Source: three-view drawing plus pictorial views. Frame: mm from the lowest corner of the part. A direction names the side the tool comes from. Give positions to 0.01 mm unless a question says otherwise; leave off trailing zeros. Order: outer loops, then holes, each group sorted by start corner. A loop starts at its lowest first (then second) coordinate and runs counter-clockwise, first axis right, second up.
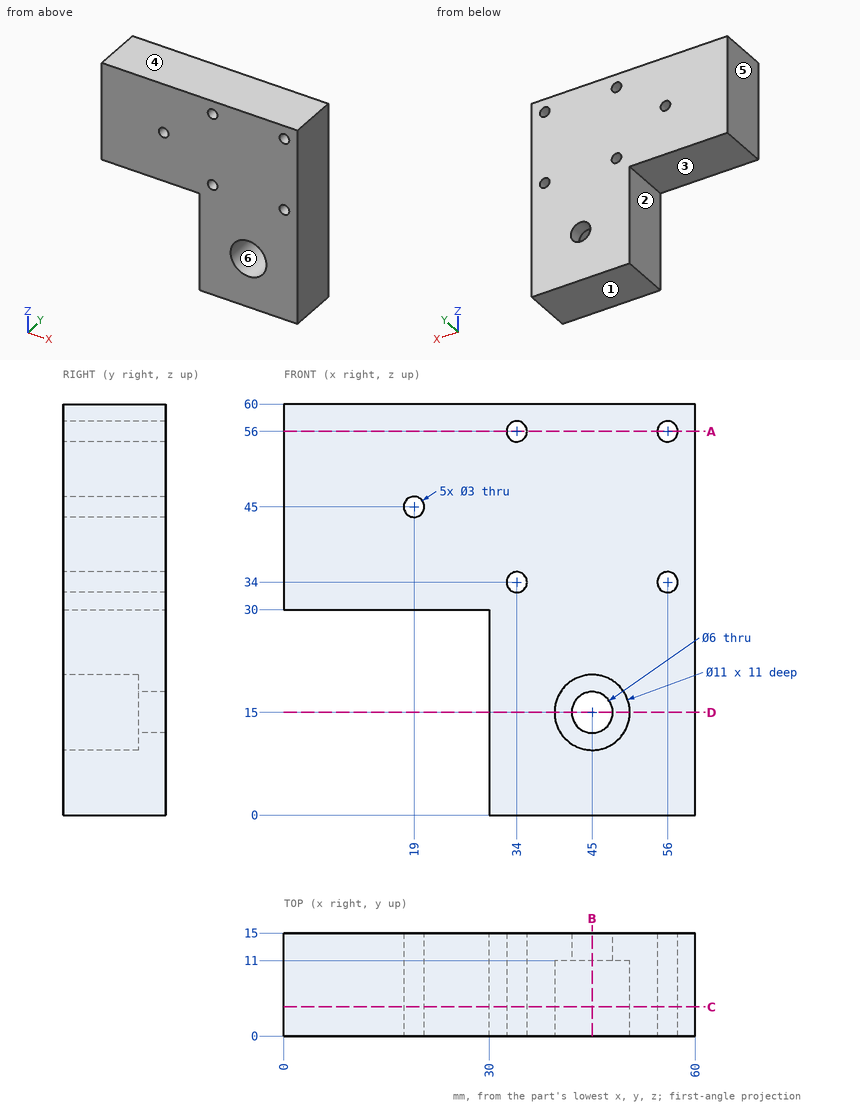
1) Reachability of the marked faces 1 and 2 from +Z, -Z, +X, -X, +Y, -Y: full face, straight path, thin tool, end or side. Return the list, or none.
Checks:
face 1: -Z, +X, -X, +Y, -Y
face 2: -Z, -X, +Y, -Y
2) Section query B-B on x = 45. Output: boundary loops of the cut face in (y, z).
Checks:
outline: (0, 0) - (15, 0) - (15, 12) - (11, 12) - (11, 9.5) - (0, 9.5) - close; (0, 20.5) - (11, 20.5) - (11, 18) - (15, 18) - (15, 60) - (0, 60) - close
3) Section query C-C on y = 4.25. Output: boundary loops of the cut face in (x, z), and give its area (3 significant figures).
Checks:
outline: (0, 30) - (30, 30) - (30, 0) - (60, 0) - (60, 60) - (0, 60) - close; hole circle Ø3 at (19, 45); hole circle Ø3 at (34, 34); hole circle Ø3 at (34, 56); hole circle Ø11 at (45, 15); hole circle Ø3 at (56, 34); hole circle Ø3 at (56, 56)
area: 2,570 mm2
4) First-contact query: pin 1 Ø1.5 at (x, y) = (26.5, 2) entering from -Z; pin 2 Ø10 at (x, z) = (45, 15) entering from -Y; pin 3 Ø6 at (y, z) = (4.5, 10) entering from -X. Flat tips, straight axial feed; report the tip coordinate or a pass-through.
Checks:
pin 1: stops at z = 30
pin 2: stops at y = 11
pin 3: stops at x = 30
5) Section query D-D on z = 15. Output: boundary loops of the cut face in (x, y), and give its area (3 significant figures).
Checks:
outline: (30, 0) - (39.5, 0) - (39.5, 11) - (42, 11) - (42, 15) - (30, 15) - close; (48, 11) - (50.5, 11) - (50.5, 0) - (60, 0) - (60, 15) - (48, 15) - close
area: 305 mm2
6) Section query A-A on z = 56. Output: boundary loops of the cut face in (x, y), and give its area (3 significant figures).
Checks:
outline: (0, 0) - (32.5, 0) - (32.5, 15) - (0, 15) - close; (35.5, 0) - (54.5, 0) - (54.5, 15) - (35.5, 15) - close; (57.5, 0) - (60, 0) - (60, 15) - (57.5, 15) - close
area: 810 mm2
7) Ray query, L1, parallel to Z at x = 56, y = 8.5; L2, parallel to X at y = 6.75, z = 57; L3, parallel to X at y = 3.25, z = 29.5. Return the intervals inside material, ascending.
Checks:
L1: z = 0 to 32.5, 35.5 to 54.5, 57.5 to 60
L2: x = 0 to 32.88, 35.12 to 54.88, 57.12 to 60
L3: x = 30 to 60
8) Pull-direction query (Z, two-part tool) for the marked faces 3, 4, 5 and 6; classes: +Z half, -Z half, draft (parallel to the pull), parting line (faces both ways), or undercut.
Checks:
face 3: -Z half
face 4: +Z half
face 5: draft
face 6: undercut
